Drawing for the job (mm, zero at the part's lowest x, y, z). A direction names the side the tool comes from. Give positions to 0.01 mm unless a question says otherwise; leave off trailing zeros. Write each loop counter-clockwise with the first axis right and the second up, starting at its lowest first coordinate (ties: lowest second). Pieces come first, ordered by that corner, then holes. Notation, with made-up numbers: M 69,26.5 L 121,26.5 A25 ccw 121,49.5 Z; hole C 47,81.25 d10. An arc over 180 degrees is marked long. Use CSV: the item, a comma, the result in double quotes. Start each with the question number.
1. Mould opens along X. For the marked faces 1, 2 and 3 say: pulls with the +X half, pulls with the -X half, needs draft (parallel to the pull), parting line crosses it, or undercut.
2. Drill centre lines: line 1 along X through (y, z) = (14, 25) (3 decimals); line 2 along X through (y, z) = (6.5, 25); line 3 along Y through (x, z) = (47, 39). Where is each one in solid material? Low to high. Write a range as from..to.
3. Drop flat-ended pins along their axis: pin 1 Ø3 at (y, z) = (21.5, 17) entering from -X; pin 2 Ø4 at (x, y) = (14.5, 22) entering from +Z; pin 3 Ø12 at (y, z) = (20, 13.5) entering from +X; pin 4 Ø10.5 at (x, z) = (25, 25) entering from -Y. Give the stop position or say it passes through.
4. Band-saw the part on A-A, the plane z = 25. List the corners of the cut face in (x, y) (3 decimals), then the cut area to 3 significant figures.
5. 3-axis set-ups, long thin cutter, end or side, ignore diameter. For the marked faces 4 and 5: which of +Z, -Z, +X, -X, +Y, -Y reach the whole face in a straight line?
6. Band-saw the part on B-B, the plane x = 25. List the corners of the cut face in (y, z) (3 decimals).
7. Band-saw the part on D-D, the plane z = 46.5. List the corners of the cut face in (x, y).
8. Band-saw the part on C-C, the plane y = 9. List the corners of the cut face in (x, z).
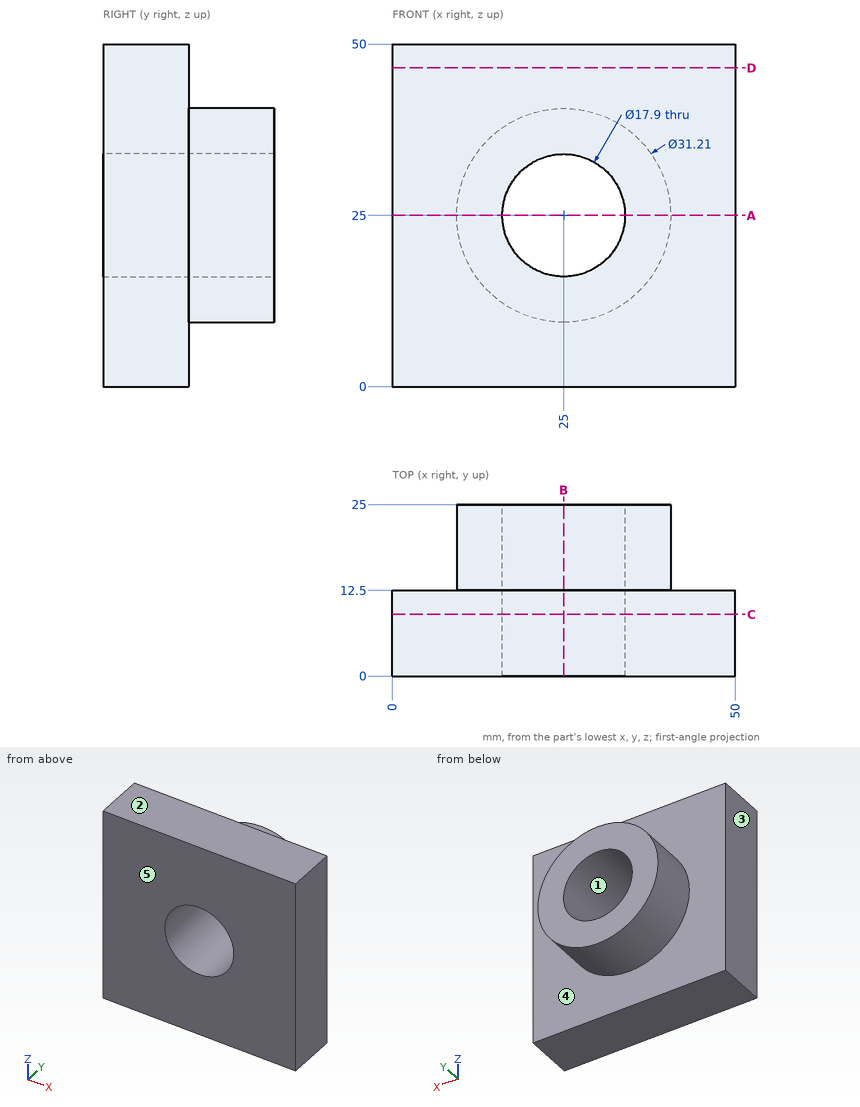
Output:
1,face 1,"undercut"
1,face 2,"needs draft"
1,face 3,"pulls with the -X half"
2,line 1,"x = 9.395..16.05, 33.95..40.605"
2,line 2,"x = 0..16.05, 33.95..50"
2,line 3,"y = 0..12.5"
3,pin 1,"stops at x = 10.81"
3,pin 2,"stops at z = 38.09"
3,pin 3,"stops at x = 39.6"
3,pin 4,"passes through"
4,outline,"M 0,0 L 16.05,0 L 16.05,25 L 9.395,25 L 9.395,12.5 L 0,12.5 Z; M 33.95,0 L 50,0 L 50,12.5 L 40.605,12.5 L 40.605,25 L 33.95,25 Z"
4,area,"568 mm²"
5,face 4,"+Y"
5,face 5,"+Z, -Z, +X, -X, -Y"
6,outline,"M 0,0 L 12.5,0 L 12.5,9.395 L 25,9.395 L 25,16.05 L 0,16.05 Z; M 0,33.95 L 25,33.95 L 25,40.605 L 12.5,40.605 L 12.5,50 L 0,50 Z"
7,outline,"M 0,0 L 50,0 L 50,12.5 L 0,12.5 Z"
8,outline,"M 0,0 L 50,0 L 50,50 L 0,50 Z; hole C 25,25 d17.9"
